Input: part model. Units: mm. Frame: model coordinates. A direction names the side the tool comes from. Coordinates: 2 decimals unless noted, no trailing zeros. Order: outer loops, then holes, each group sorted by start corner. A loop starts at its lowest first (then second) coordinate and runs counter-clockwise, first axis right, second up. Notation, with made-up numbers: M 75.5,-33 L 127.5,-33 A15 ccw 127.5,-12 Z; hole C 37.5,31.5 d4. An arc over 180 degrees is marked long. One line per item, written item: value.
```python
from build123d import *

# Parameters (mm, degrees)
SKETCH_1_R               = 8
EXTRUDE_1_DEPTH          = 51
SKETCH_2_R               = 7
CUT_EXTRUDE_1_DEPTH      = 38
CUT_EXTRUDE_2_DEPTH      = 53.239831546
CUT_EXTRUDE_2_DEPTH_BACK = 53.239831546
SKETCH_3_W               = 2.2
SKETCH_3_H               = 22
FILLET_1_R               = 0.5
FILLET_2_R               = 1
SKETCH_4_R               = 3
CUT_EXTRUDE_3_DEPTH      = 53.239831675
SKETCH_5_R               = 1.5
CUT_EXTRUDE_8_DEPTH      = 38


with BuildPart() as part:
    # 草图1 → 凸台-拉伸1 (new body)
    with BuildSketch(Plane(origin=(0, 0, 0), x_dir=(1, 0, 0), z_dir=(0, 1, 0))):
        with Locations(Location((0, 0, 0), (0, 0, 270))):
            Circle(SKETCH_1_R)
    extrude(amount=EXTRUDE_1_DEPTH)

    # 草图2 → 切除-拉伸1 (cut)
    with BuildSketch(Plane(origin=(0, 51, 0), x_dir=(1, 0, 0), z_dir=(0, 1, 0))):
        with Locations(Location((0, 0, 0), (0, 0, 270))):
            Circle(SKETCH_2_R)
    extrude(amount=-CUT_EXTRUDE_1_DEPTH, mode=Mode.SUBTRACT)

    # 草图3 → 切除-拉伸2 (cut, two sides: drawn at the far end of the back side and taken through both)
    with BuildSketch(Plane(origin=(0, 0, 0), x_dir=(0, 0, -1), z_dir=(1, 0, 0)).offset(-CUT_EXTRUDE_2_DEPTH_BACK)):
        with Locations((0, 51)):
            Rectangle(SKETCH_3_W, SKETCH_3_H)
    extrude(amount=CUT_EXTRUDE_2_DEPTH + CUT_EXTRUDE_2_DEPTH_BACK, mode=Mode.SUBTRACT)

    # 圆角1
    fillet_1_edges = [part.edges().sort_by_distance(p)[0] for p in [
        (7.418522654, 51, -1.1),
        (-7.418522654, 51, -1.1),
        (-7.418522654, 51, 1.1),
        (7.418522654, 51, 1.1),
    ]]
    fillet(fillet_1_edges, radius=FILLET_1_R)

    # 圆角2
    fillet_2_edges = [part.edges().sort_by_distance(p)[0] for p in [
        (7.418522654, 40, -1.1),
        (-7.418522654, 40, -1.1),
        (7.418522654, 40, 1.1),
        (-7.418522654, 40, 1.1),
    ]]
    fillet(fillet_2_edges, radius=FILLET_2_R)

    # 草图4 → 切除-拉伸3 (cut, through all)
    with BuildSketch(Plane(origin=(0, 0, 0), x_dir=(-1, 0, 0), z_dir=(0, -1, 0))):
        with Locations(Location((0, 0, 0), (0, 0, 90))):
            Circle(SKETCH_4_R)
    extrude(amount=-CUT_EXTRUDE_3_DEPTH, mode=Mode.SUBTRACT)

    # 草图5 → 切除-拉伸8 (cut)
    with BuildSketch(Plane.XZ):
        with Locations(Location((0, 5.5, 0), (0, 0, 270))):
            Circle(SKETCH_5_R)
    extrude(amount=-CUT_EXTRUDE_8_DEPTH, mode=Mode.SUBTRACT)


solid = part.part
```
(1) First-contact query: pin 1 (6 mm diameter, centred on y = 22, z = 4, fed in from +X); pin 2 (2.5 mm diameter, centred on x = 0, z = 5.5, fed in from +Y); pin 3 (1.1 mm diameter, centred on x = 7.5, y = 44, fed in from -Z); pin 4 (0.8 mm diameter, centred on x = 7.5, y = 44, fed in from +Z). Flat tips, straight axial feed; report the tip coordinate or a pass-through.
Data:
pin 1: stops at x = 7.94
pin 2: passes through
pin 3: stops at z = -3.96
pin 4: stops at z = 3.69
(2) Cut plane A-A on y = 45. Output: boundary loops of the cut face in (x, z), plus the area to 3 significant figures.
Data:
outline: M -7.92,-1.1 A8 ccw 7.92,-1.1 L 6.91,-1.1 A7 cw -6.91,-1.1 Z; M -7.92,1.1 L -6.91,1.1 A7 cw 6.91,1.1 L 7.92,1.1 A8 ccw Z
area: 42.7 mm2
(3) Access query for faces 1 (the cylindrical face through (-6.834, 32.266, -1.517)), 2 (the flat face through (0, 51, 7.2)), 3 (the cylindrical face through (7.464, 40.285, -0.799)). Directions: +Z, -Z, +X, -X, +Y, -Y. A direction counts if a zero-diameter tool reaches every point of the face in a straight line with its end or side. Return the directions, or none.
Data:
face 1: +Y
face 2: +Z, -Z, +X, -X, +Y
face 3: +X, -X, +Y
(4) Cut plane C-C on x = -1. Output: boundary loops of the cut face in (y, z).
Data:
outline: M 0,-7.94 L 51,-7.94 L 51,-6.93 L 13,-6.93 L 13,-2.83 L 0,-2.83 Z; M 0,2.83 L 13,2.83 L 13,4.38 L 0,4.38 Z; M 0,6.62 L 13,6.62 L 13,6.93 L 51,6.93 L 51,7.94 L 0,7.94 Z
(5) Cut plane B-B on z = 2.5. Output: boundary loops of the cut face in (x, y).
Data:
outline: M -7.6,0 L -1.66,0 L -1.66,13 L -6.54,13 L -6.54,51 L -7.6,51 Z; M 1.66,0 L 7.6,0 L 7.6,51 L 6.54,51 L 6.54,13 L 1.66,13 Z
(6) Cut plane D-D on x = 5.5. Output: boundary loops of the cut face in (y, z), plus the area to 3 significant figures.
Data:
outline: M 0,-5.81 L 51,-5.81 L 51,-4.33 L 13,-4.33 L 13,4.33 L 51,4.33 L 51,5.81 L 0,5.81 Z
area: 263 mm2
(7) Ray query, line 1 (X direction, y = 5.5, z = 0); line 2 (X direction, y = 37, z = 0); line 3 (Z direction, x = -3, y = 41). Return the intervals inside material, ascending. Write a range as from..to.
Data:
line 1: x = -8..-3, 3..8
line 2: x = -8..-7, 7..8
line 3: z = -7.42..-6.32, 6.32..7.42
(8) Draft query along X for faces 4 (the cylindrical face through (0.9, 6.41, -2.86)), 5 (the flat face through (0, 51, -7.2)), 6 (the cylindrical face through (-7.81, 25.14, -1.73)), 7 (the cylindrical face through (0, 6, 7)). Return one class per face: released by +X, released by -X, zero draft, split by the parting line, or undercut.
Data:
face 4: undercut
face 5: zero draft
face 6: split by the parting line
face 7: undercut
